Drawing for the job (mm, zero at the part's lowest x, y, z). A direction names the side the tool comes from. Give positions to 0.01 mm unless a question says otherwise; leave off trailing zeros. Write each loop counter-clockwise with the first axis right and the second up, starting at its lowest first coordinate (ties: lowest second). Pieces come first, ordered by that corner, then holes.
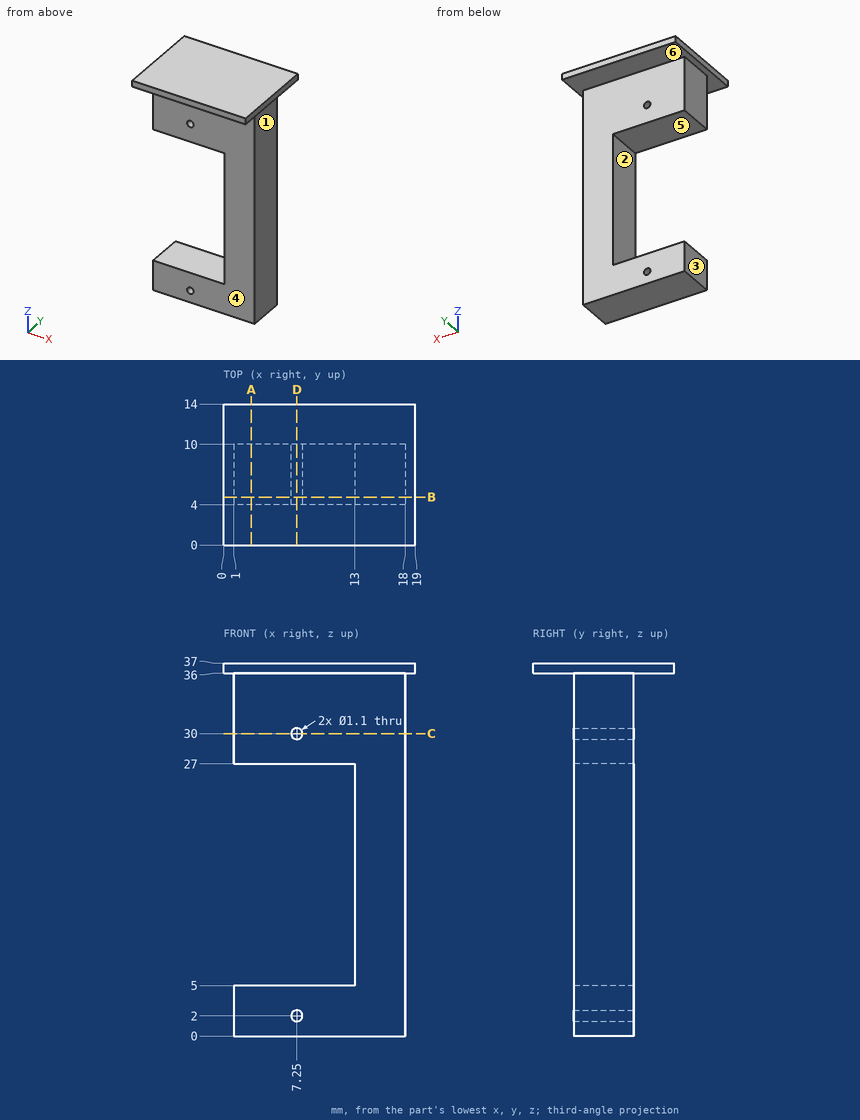
1. Slice it at B-B, the plane y = 4.75. Write the cut outline in (x, z).
Calculated:
outline: (0, 36) - (1, 36) - (1, 27) - (13, 27) - (13, 5) - (1, 5) - (1, 0) - (18, 0) - (18, 36) - (19, 36) - (19, 37) - (0, 37) - close; hole circle Ø1.1 at (7.25, 2); hole circle Ø1.1 at (7.25, 30)
2. Slice it at D-D, the plane x = 7.25. Write the cut outline in (y, z).
Calculated:
outline: (0, 36) - (4, 36) - (4, 30.55) - (10, 30.55) - (10, 36) - (14, 36) - (14, 37) - (0, 37) - close; (4, 0) - (10, 0) - (10, 1.45) - (4, 1.45) - close; (4, 2.55) - (10, 2.55) - (10, 5) - (4, 5) - close; (4, 27) - (10, 27) - (10, 29.45) - (4, 29.45) - close
3. Pin check, flat tips, straight feed: P1, Ø8, axis at x = 9, z = 24.5, coming from the -Y side; P2, Ø1, axis at x = 7, y = 1.5, coming from the -Z side; P3, Ø3, axis at x = 10, y = 5, coming from the -Z side; P4, Ø1, axis at y = 7, z = 30.5, coming from the -X side. Stop position of each tip, or through.
Calculated:
P1: stops at y = 4
P2: stops at z = 36
P3: stops at z = 0
P4: stops at x = 1
4. Which spindle directions (+Z, -Z, +X, -X, +Y, -Y) get a long thin tool onto all of the face, cutting with end or side? Do the marked faces 1, 2 and 3. Say none if no direction does.
Calculated:
face 1: -Z, +X, +Y, -Y
face 2: -X, +Y, -Y
face 3: -Z, -X, +Y, -Y
5. Probe probe 1 along Z at (x, y) = (7.25, 7.45); probe 2 along Z at (x, y) = (4, 13.25); probe 3 along Y at (x, z) = (3.5, 34). List the from-to ranges inside material, lowest first.
Calculated:
probe 1: z = 0 to 1.45, 2.55 to 5, 27 to 29.45, 30.55 to 37
probe 2: z = 36 to 37
probe 3: y = 4 to 10
6. Pull direction Z, two halves, no side cores. Call the marked faces 4, 5 and 6: +Z half, -Z half, draft (parallel to the pull), parting line (faces both ways), or undercut.
Calculated:
face 4: draft
face 5: undercut
face 6: -Z half
7. Slice it at C-C, the plane z = 30. Write the cut outline in (x, y), and give its area (3 significant figures).
Calculated:
outline: (1, 4) - (6.7, 4) - (6.7, 10) - (1, 10) - close; (7.8, 4) - (18, 4) - (18, 10) - (7.8, 10) - close
area: 95.4 mm2
8. Slice it at A-A, the plane x = 2.75. Write the cut outline in (y, z).
Calculated:
outline: (0, 36) - (4, 36) - (4, 27) - (10, 27) - (10, 36) - (14, 36) - (14, 37) - (0, 37) - close; (4, 0) - (10, 0) - (10, 5) - (4, 5) - close
